from build123d import *

# Parameters (mm, degrees)
F0_R     = 10.7188
F1_DEPTH = 12.3952
F2_W     = 38.1
F2_H     = 12.3952
F3_DEPTH = 9.2964
F4_W     = 12.3952
F4_H     = 38.1
F5_DEPTH = 12.3952


with BuildPart() as f1:
    # F0 (on Top) → F1 (new body)
    with BuildSketch(Plane.XY):
        Polygon((370.379505, 441.401105), (0, 0), (584.2, 0), align=None)
        with Locations((370.379505, 99.24288)):
            Circle(F0_R, mode=Mode.SUBTRACT)
        with Locations((370.379505, 213.868)):
            Circle(F0_R, mode=Mode.SUBTRACT)
        with Locations((370.379505, 370.332)):
            Circle(F0_R, mode=Mode.SUBTRACT)
    extrude(amount=F1_DEPTH)

    # F2 (on face) → F3 (join)
    with BuildSketch(Plane.XZ):
        with Locations((57.15, 6.1976)):
            Rectangle(F2_W, F2_H)
        with Locations((292.1, 6.1976)):
            Rectangle(F2_W, F2_H)
        with Locations((527.05, 6.1976)):
            Rectangle(F2_W, F2_H)
    extrude(amount=F3_DEPTH)

    # F4 (on face) → F5 (cut, through all)
    with BuildSketch(Plane(origin=(0, 0, 0), x_dir=(1, 0, 0), z_dir=(0, 0, -1))):
        with Locations((415.294277, -70.7644)):
            Rectangle(F4_W, F4_H)
        with Locations((327.003877, -70.7644)):
            Rectangle(F4_W, F4_H)
        with Locations((238.713477, -70.7644)):
            Rectangle(F4_W, F4_H)
        with Locations((175.823077, -70.7644)):
            Rectangle(F4_W, F4_H)
    extrude(amount=-F5_DEPTH, mode=Mode.SUBTRACT)


solid = f1.part
Work out the finished part from the listing and answer in its coordinate system (mm). A direction names the side the tool comes from. Give positions to 0.01 mm unless a question says otherwise; leave off trailing zeros. Write each loop counter-clockwise with the first axis right and the second up, starting at its lowest first coordinate (ties: lowest second). Pieces come first, ordered by that corner, then holes.
Q1. The part is cut by section C-C on y = 290. Give the vertices of the cut face in (x, z), and give its area (3 significant figures).
Answer:
outline: (243.34, 0) - (443.72, 0) - (443.72, 12.4) - (243.34, 12.4) - close
area: 2,480 mm2
Q2. A tool of negligible diameter and unlimited length cuts with its end or side. For faces 1 (the face through (57, -9.296, 6)), 2 (the face through (173, 0, 6)), 3 (the face through (288, 169, 0)), 4 (the face through (320.806, 71, 6)), 5 (the face through (19, 0, 6)), from which of +Z, -Z, +X, -X, +Y, -Y can it reach the whole face along a straight path? Write none if from no direction.
Answer:
face 1: +Z, -Z, +X, -X, -Y
face 2: +Z, -Z, -Y
face 3: -Z, +X, -X, +Y, -Y
face 4: +Z, -Z
face 5: +Z, -Z, -X, -Y
Q3. The part is cut by section B-B on x = 188. Give the vertices of the cut face in (y, z), and give its area (3 significant figures).
Answer:
outline: (0, 0) - (224.05, 0) - (224.05, 12.4) - (0, 12.4) - close
area: 2,780 mm2
Q4. Given pin 1 (3 mm diameter, centred on y = -3, z = 6, fed in from +X); pin 2 (1.5 mm diameter, centred on y = 322.5, z = 4, fed in from +X); pin 3 (3.5 mm diameter, centred on y = 77.5, z = 5.5, fed in from -X), each flat-ended and moving along its own axis, determine where each tip first touches the part or whether it passes through.
Answer:
pin 1: stops at x = 546.1
pin 2: stops at x = 428.34
pin 3: stops at x = 63.56
Q5. For a pull along Y with two mould halves and no side action, classify faces 6 (the face through (409.097, 71, 6)), 7 (the face through (187.78, 223.79, 6.11)), 8 (the face through (415, 51.714, 6)), 9 (the face through (408, 0, 6)) as released by +Y, released by -Y, zero draft, split by the parting line, or undercut.
Answer:
face 6: undercut
face 7: released by +Y
face 8: undercut
face 9: released by -Y
Q6. Straight lines are drawn through the part: L1, parallel to Y at x = 361, z = 2; L2, parallel to X at y = 93.5, z = 3.75; L3, parallel to X at y = 361.5, z = 4.75. For each, find the intervals that lie inside material, in ascending order.
Answer:
L1: y = 0 to 94.05, 104.43 to 208.68, 219.06 to 365.14, 375.52 to 430.22
L2: x = 78.46 to 361.33, 379.43 to 538.91
L3: x = 303.33 to 364.31, 376.45 to 409.08
Q7. The part is cut by section A-A on z = 9.75. State how many separate pieces and enclosed holes the cut face has, and give its area (3 significant figures).
Answer:
separate pieces: 1
enclosed holes: 7
area: 127,000 mm2
